```python
from build123d import *

# Parameters (mm, degrees)
SKETCH1_W           = 30
SKETCH1_H           = 30
BOSS_EXTRUDE1_DEPTH = 12
SKETCH2_W           = 12
SKETCH2_H           = 25
BOSS_EXTRUDE2_DEPTH = 40.5
SKETCH3_R           = 1.6
CUT_EXTRUDE1_DEPTH  = 10
FILLET1_R           = 10


with BuildPart() as part:
    # Sketch1 → Boss-Extrude1 (new body)
    with BuildSketch(Plane(origin=(0, 0, 0), x_dir=(1, 0, 0), z_dir=(0, 1, 0))):
        Rectangle(SKETCH1_W, SKETCH1_H)
    extrude(amount=BOSS_EXTRUDE1_DEPTH)

    # Sketch2 → Boss-Extrude2 (add)
    with BuildSketch(Plane(origin=(0, 12, 0), x_dir=(1, 0, 0), z_dir=(0, 1, 0))):
        Rectangle(SKETCH2_W, SKETCH2_H)
    extrude(amount=BOSS_EXTRUDE2_DEPTH)

    # Sketch3 → Cut-Extrude1 (cut)
    with BuildSketch(Plane(origin=(0, 52.5, 0), x_dir=(1, 0, 0), z_dir=(0, 1, 0))):
        with Locations(Location((0, -7.5, 0), (0, 0, 270))):
            Circle(SKETCH3_R)
        with Locations(Location((0, 7.5, 0), (0, 0, 270))):
            Circle(SKETCH3_R)
    extrude(amount=-CUT_EXTRUDE1_DEPTH, mode=Mode.SUBTRACT)

    # Fillet1
    # the kernel refuses this fillet: 10 mm, written as the material it adds along each edge
    with BuildSketch(Plane(origin=(6, 12, 12.5), x_dir=(1, 0, 0), z_dir=(0, 0, -1)), Plane(origin=(-6, 12, -12.5), x_dir=(-1, 0, 0), z_dir=(0, 0, 1))) as fillet1_piece_1:
        with BuildLine():
            CenterArc((10, -9.949874371), FILLET1_R, 95.739170477, 84.260829523)
            Line((0, -9.949874371), (-0.2, -9.949874371))
            Line((-0.2, -9.949874371), (-0.2, 0))
            Line((-0.2, 0), (0, 0.2))
            ThreePointArc((0, 0.2), (4.5, 0.2), (8.98, 0.198997487))
            Line((8.98, 0.198997487), (9, 0))
        make_face()
    extrude(amount=25)
    with BuildSketch(Plane(origin=(6, 12, -12.5), x_dir=(0, 0, -1), z_dir=(-1, 0, 0)), Plane(origin=(-6, 12, 12.5), x_dir=(0, 0, 1), z_dir=(1, 0, 0))) as fillet1_piece_2:
        with BuildLine():
            CenterArc((10, -6.614378278), FILLET1_R, 138.590377891, 41.409622109)
            Line((0, -6.614378278), (-0.2, -6.614378278))
            Line((-0.2, -6.614378278), (-0.2, 0))
            Line((-0.2, 0), (0, 0.2))
            ThreePointArc((0, 0.2), (1.25, 0.2), (2.35, 0.132287566))
            Line((2.35, 0.132287566), (2.5, 0))
        make_face()
    extrude(amount=12)
    with BuildSketch(Plane(origin=(6, 12, 37.374685928), x_dir=(1, 0, 0), z_dir=(0, 0, -1))) as fillet1_piece_3a_section:
        with BuildLine():
            CenterArc((10, -9.949874371), FILLET1_R, 95.739170477, 84.260829523)
            Line((0, -9.949874371), (-0.2, -9.949874371))
            Line((-0.2, -9.949874371), (-0.2, 0))
            Line((-0.2, 0), (0, 0.2))
            ThreePointArc((0, 0.2), (4.5, 0.2), (8.98, 0.198997487))
            Line((8.98, 0.198997487), (9, 0))
        make_face()
    fillet1_piece_3a = extrude(amount=49.874685928, mode=Mode.PRIVATE)
    fillet1_piece_3a = split(fillet1_piece_3a, bisect_by=Plane(origin=(8.162151556, 14.281986067, 15), z_dir=(0, 0, -1)), keep=Keep.TOP, mode=Mode.PRIVATE)
    fillet1_piece_3a = split(fillet1_piece_3a, bisect_by=Plane(origin=(8.162151556, 14.281986067, 12.5), z_dir=(0, 0, 1)), keep=Keep.TOP, mode=Mode.PRIVATE)
    with BuildSketch(Plane(origin=(-6, 12, 12.5), x_dir=(0, 0, 1), z_dir=(1, 0, 0))) as fillet1_piece_3b_section:
        with BuildLine():
            CenterArc((10, -6.614378278), FILLET1_R, 138.590377891, 41.409622109)
            Line((0, -6.614378278), (-0.2, -6.614378278))
            Line((-0.2, -6.614378278), (-0.2, 0))
            Line((-0.2, 0), (0, 0.2))
            ThreePointArc((0, 0.2), (1.25, 0.2), (2.35, 0.132287566))
            Line((2.35, 0.132287566), (2.5, 0))
        make_face()
    fillet1_piece_3b = extrude(amount=28.535945694, mode=Mode.PRIVATE)
    fillet1_piece_3b = split(fillet1_piece_3b, bisect_by=Plane(origin=(15, 13.814075663, 13.097749904), z_dir=(-1, 0, 0)), keep=Keep.TOP, mode=Mode.PRIVATE)
    fillet1_piece_3b = split(fillet1_piece_3b, bisect_by=Plane(origin=(6, 13.814075663, 13.097749904), z_dir=(1, 0, 0)), keep=Keep.TOP, mode=Mode.PRIVATE)
    fillet1_piece_3 = fillet1_piece_3a & fillet1_piece_3b
    add(fillet1_piece_3)
    with BuildSketch(Plane(origin=(6, 12, 12.5), x_dir=(1, 0, 0), z_dir=(0, 0, -1))) as fillet1_piece_4a_section:
        with BuildLine():
            CenterArc((10, -9.949874371), FILLET1_R, 95.739170477, 84.260829523)
            Line((0, -9.949874371), (-0.2, -9.949874371))
            Line((-0.2, -9.949874371), (-0.2, 0))
            Line((-0.2, 0), (0, 0.2))
            ThreePointArc((0, 0.2), (4.5, 0.2), (8.98, 0.198997487))
            Line((8.98, 0.198997487), (9, 0))
        make_face()
    fillet1_piece_4a = extrude(amount=49.874685928, mode=Mode.PRIVATE)
    fillet1_piece_4a = split(fillet1_piece_4a, bisect_by=Plane(origin=(8.162151556, 14.281986067, -15), z_dir=(0, 0, 1)), keep=Keep.TOP, mode=Mode.PRIVATE)
    fillet1_piece_4a = split(fillet1_piece_4a, bisect_by=Plane(origin=(8.162151556, 14.281986067, -12.5), z_dir=(0, 0, -1)), keep=Keep.TOP, mode=Mode.PRIVATE)
    with BuildSketch(Plane(origin=(22.535945694, 12, -12.5), x_dir=(0, 0, -1), z_dir=(-1, 0, 0))) as fillet1_piece_4b_section:
        with BuildLine():
            CenterArc((10, -6.614378278), FILLET1_R, 138.590377891, 41.409622109)
            Line((0, -6.614378278), (-0.2, -6.614378278))
            Line((-0.2, -6.614378278), (-0.2, 0))
            Line((-0.2, 0), (0, 0.2))
            ThreePointArc((0, 0.2), (1.25, 0.2), (2.35, 0.132287566))
            Line((2.35, 0.132287566), (2.5, 0))
        make_face()
    fillet1_piece_4b = extrude(amount=28.535945694, mode=Mode.PRIVATE)
    fillet1_piece_4b = split(fillet1_piece_4b, bisect_by=Plane(origin=(15, 13.814075663, -13.097749904), z_dir=(-1, 0, 0)), keep=Keep.TOP, mode=Mode.PRIVATE)
    fillet1_piece_4b = split(fillet1_piece_4b, bisect_by=Plane(origin=(6, 13.814075663, -13.097749904), z_dir=(1, 0, 0)), keep=Keep.TOP, mode=Mode.PRIVATE)
    fillet1_piece_4 = fillet1_piece_4a & fillet1_piece_4b
    add(fillet1_piece_4)
    with BuildSketch(Plane(origin=(-6, 12, -37.374685928), x_dir=(-1, 0, 0), z_dir=(0, 0, 1))) as fillet1_piece_5a_section:
        with BuildLine():
            CenterArc((10, -9.949874371), FILLET1_R, 95.739170477, 84.260829523)
            Line((0, -9.949874371), (-0.2, -9.949874371))
            Line((-0.2, -9.949874371), (-0.2, 0))
            Line((-0.2, 0), (0, 0.2))
            ThreePointArc((0, 0.2), (4.5, 0.2), (8.98, 0.198997487))
            Line((8.98, 0.198997487), (9, 0))
        make_face()
    fillet1_piece_5a = extrude(amount=49.874685928, mode=Mode.PRIVATE)
    fillet1_piece_5a = split(fillet1_piece_5a, bisect_by=Plane(origin=(-8.162151556, 14.281986067, -15), z_dir=(0, 0, 1)), keep=Keep.TOP, mode=Mode.PRIVATE)
    fillet1_piece_5a = split(fillet1_piece_5a, bisect_by=Plane(origin=(-8.162151556, 14.281986067, -12.5), z_dir=(0, 0, -1)), keep=Keep.TOP, mode=Mode.PRIVATE)
    with BuildSketch(Plane(origin=(6, 12, -12.5), x_dir=(0, 0, -1), z_dir=(-1, 0, 0))) as fillet1_piece_5b_section:
        with BuildLine():
            CenterArc((10, -6.614378278), FILLET1_R, 138.590377891, 41.409622109)
            Line((0, -6.614378278), (-0.2, -6.614378278))
            Line((-0.2, -6.614378278), (-0.2, 0))
            Line((-0.2, 0), (0, 0.2))
            ThreePointArc((0, 0.2), (1.25, 0.2), (2.35, 0.132287566))
            Line((2.35, 0.132287566), (2.5, 0))
        make_face()
    fillet1_piece_5b = extrude(amount=28.535945694, mode=Mode.PRIVATE)
    fillet1_piece_5b = split(fillet1_piece_5b, bisect_by=Plane(origin=(-15, 13.814075663, -13.097749904), z_dir=(1, 0, 0)), keep=Keep.TOP, mode=Mode.PRIVATE)
    fillet1_piece_5b = split(fillet1_piece_5b, bisect_by=Plane(origin=(-6, 13.814075663, -13.097749904), z_dir=(-1, 0, 0)), keep=Keep.TOP, mode=Mode.PRIVATE)
    fillet1_piece_5 = fillet1_piece_5a & fillet1_piece_5b
    add(fillet1_piece_5)
    with BuildSketch(Plane(origin=(-22.535945694, 12, 12.5), x_dir=(0, 0, 1), z_dir=(1, 0, 0))) as fillet1_piece_6a_section:
        with BuildLine():
            CenterArc((10, -6.614378278), FILLET1_R, 138.590377891, 41.409622109)
            Line((0, -6.614378278), (-0.2, -6.614378278))
            Line((-0.2, -6.614378278), (-0.2, 0))
            Line((-0.2, 0), (0, 0.2))
            ThreePointArc((0, 0.2), (1.25, 0.2), (2.35, 0.132287566))
            Line((2.35, 0.132287566), (2.5, 0))
        make_face()
    fillet1_piece_6a = extrude(amount=28.535945694, mode=Mode.PRIVATE)
    fillet1_piece_6a = split(fillet1_piece_6a, bisect_by=Plane(origin=(-15, 13.814075663, 13.097749904), z_dir=(1, 0, 0)), keep=Keep.TOP, mode=Mode.PRIVATE)
    fillet1_piece_6a = split(fillet1_piece_6a, bisect_by=Plane(origin=(-6, 13.814075663, 13.097749904), z_dir=(-1, 0, 0)), keep=Keep.TOP, mode=Mode.PRIVATE)
    with BuildSketch(Plane(origin=(-6, 12, -12.5), x_dir=(-1, 0, 0), z_dir=(0, 0, 1))) as fillet1_piece_6b_section:
        with BuildLine():
            CenterArc((10, -9.949874371), FILLET1_R, 95.739170477, 84.260829523)
            Line((0, -9.949874371), (-0.2, -9.949874371))
            Line((-0.2, -9.949874371), (-0.2, 0))
            Line((-0.2, 0), (0, 0.2))
            ThreePointArc((0, 0.2), (4.5, 0.2), (8.98, 0.198997487))
            Line((8.98, 0.198997487), (9, 0))
        make_face()
    fillet1_piece_6b = extrude(amount=49.874685928, mode=Mode.PRIVATE)
    fillet1_piece_6b = split(fillet1_piece_6b, bisect_by=Plane(origin=(-8.162151556, 14.281986067, 15), z_dir=(0, 0, -1)), keep=Keep.TOP, mode=Mode.PRIVATE)
    fillet1_piece_6b = split(fillet1_piece_6b, bisect_by=Plane(origin=(-8.162151556, 14.281986067, 12.5), z_dir=(0, 0, 1)), keep=Keep.TOP, mode=Mode.PRIVATE)
    fillet1_piece_6 = fillet1_piece_6a & fillet1_piece_6b
    add(fillet1_piece_6)


solid = part.part
```
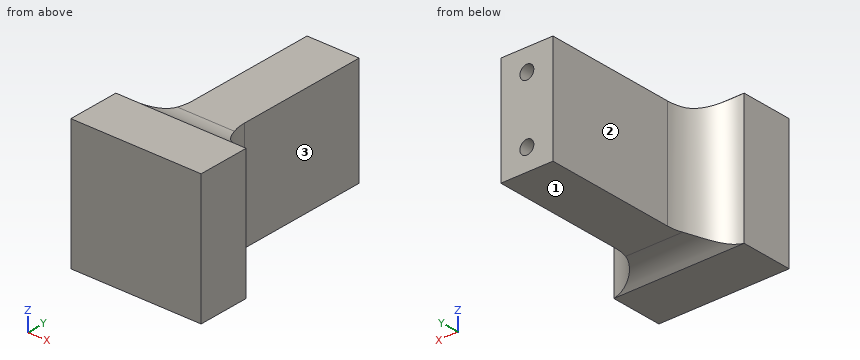
Check sheet for the modelled part. Datum: model origin and axes. Units: mm. Face numbers are marked on the shaded views. A direction names the side the tool comes from. Coordinates: 2 decimals unless noted, no trailing zeros. Order: outer loops, then holes, each group sorted by start corner. A loop starts at its lowest first (then second) coordinate and runs counter-clockwise, first axis right, second up. Notation, with made-up numbers: (74, 83) -> (103, 83) arc R19 ccw to (103, 115) -> close; hole circle Ø6 at (15, 89.5). An arc over 180 degrees is marked (long way). Write each question's results on one line, items separated by ' | '. Start each with the question number.
1) Section check C-C (z = 7.5). Enter the section's corners in (x, y), and give its area (3 significant figures).
2) Section check D-D (y = 32.5). Enter the section's corners in (x, z).
3) Set-up check for the marked faces 1, 2 and 3: record each of +Z, -Z, +X, -X, +Y, -Y from which the full face is reachable in a straight line by a thin tool's end or side.
4) Material ranges on line 1 along X through (y, z) = (49, -7.5); line 2 along X through (y, z) = (48, -7); line 3 along X through (y, z) = (30, 2.5), recorded low to high.
5) Section check A-A (z = -2.5). Enter the section's corners in (x, y).
6) Depth check by flat-ended pin: pin 1 (1 mm diameter, centred on x = 0.5, z = -7, fed in from +Y); pin 2 (1 mm diameter, centred on x = 9, z = -2.5, fed in from +Y); pin 3 (12.5 mm diameter, centred on y = 40, z = 2.5, fed in from +X); pin 4 (1.9 mm diameter, centred on x = 0, z = 7.5, fed in from -Y). Enter the tip coordinate at first touch or a pass-through.
7) Section check B-B (x = 3). Enter the section's corners in (y, z), and give its area (3 significant figures).
Checked values:
1) outline: (-15, 0) -> (15, 0) -> (15, 12) arc R10 cw to (6, 21.95) -> (6, 52.5) -> (1.6, 52.5) -> (1.6, 42.5) -> (-1.6, 42.5) -> (-1.6, 52.5) -> (-6, 52.5) -> (-6, 21.95) arc R10 cw to (-15, 12) -> close | area: 856 mm²
2) outline: (-6, -12.5) -> (6, -12.5) -> (6, 12.5) -> (-6, 12.5) -> close
3) face 1: -Z, +X, -X, +Y | face 2: +Z, -Z, -X, +Y | face 3: +Z, -Z, +X, +Y
4) line 1: -6 to -1.6, 1.6 to 6 | line 2: -6 to -1.52, 1.52 to 6 | line 3: -6 to 6
5) outline: (-15, 0) -> (15, 0) -> (15, 12) arc R10 cw to (6, 21.95) -> (6, 52.5) -> (-6, 52.5) -> (-6, 21.95) arc R10 cw to (-15, 12) -> close
6) pin 1: y = 42.5 | pin 2: y = 15.34 | pin 3: x = 6 | pin 4: y = 0
7) outline: (0, -15) -> (12, -15) arc R10 cw to (18.61, -12.5) -> (52.5, -12.5) -> (52.5, 12.5) -> (18.61, 12.5) arc R10 cw to (12, 15) -> (0, 15) -> close | area: 1,380 mm²
